Verification items for the finished model (mm, model axes). Coordinates: 2 decimals unless noted, no trailing zeros. Write each loop counter-clockwise with the first axis right and the second up, starting at its lowest first coordinate (ties: lowest second). Pieces come first, ordered by that corner, then holes. Notation, with made-up numbers: (49.25, 30.5) -> (106.25, 30.5) arc R20 ccw to (106.25, 59.5) -> close; hole circle Ø4 at (-18.75, -2.5). An arc over 180 degrees is marked (long way). Answer in a Markdown table with one row per item.
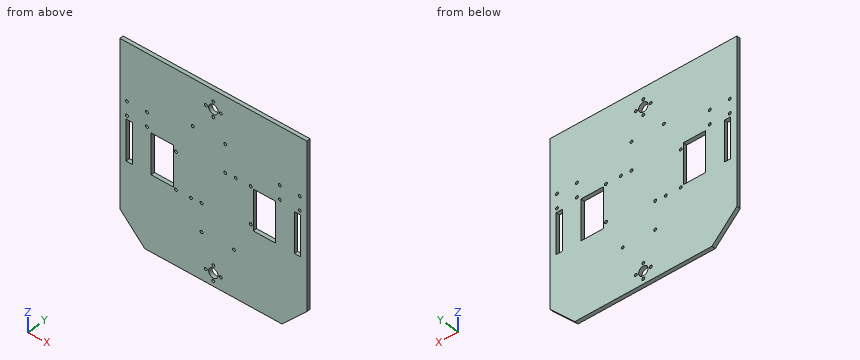
```python
from build123d import *

# Parameters (mm, degrees)
ESQUISSE1_R              = 7.5
ESQUISSE1_R_2            = 2.3
BOSS_EXTRU_1_DEPTH       = 6
ESQUISSE7_W              = 10
ESQUISSE7_H              = 64
ENL_V_MAT_EXTRU_9_DEPTH  = 10.5
ESQUISSE6_R              = 2.3
ENL_V_MAT_EXTRU_10_DEPTH = 50
ENL_V_MAT_EXTRU_11_DEPTH = 50
ESQUISSE11_R             = 2.3
ENL_V_MAT_EXTRU_15_DEPTH = 10


with BuildPart() as part:
    # Esquisse1 → Boss.-Extru.1 (new body)
    with BuildSketch(Plane(origin=(0, 0, 0), x_dir=(1, 0, 0), z_dir=(0, 1, 0))):
        Polygon((-150, 0), (-150, 260), (-110, 300), (110, 300), (150, 260), (150, 0), align=None)
        with Locations(Location((0, 30, 0), (0, 0, 270))):
            Circle(ESQUISSE1_R, mode=Mode.SUBTRACT)
        with Locations(Location((0, 18, 0), (0, 0, 270))):
            Circle(ESQUISSE1_R_2, mode=Mode.SUBTRACT)
        with Locations(Location((12, 30, 0), (0, 0, 270))):
            Circle(ESQUISSE1_R_2, mode=Mode.SUBTRACT)
        with Locations(Location((0, 42, 0), (0, 0, 270))):
            Circle(ESQUISSE1_R_2, mode=Mode.SUBTRACT)
        with Locations(Location((-12, 30, 0), (0, 0, 270))):
            Circle(ESQUISSE1_R_2, mode=Mode.SUBTRACT)
        with Locations(Location((0, 280, 0), (0, 0, 270))):
            Circle(ESQUISSE1_R, mode=Mode.SUBTRACT)
        with Locations(Location((-12, 280, 0), (0, 0, 270))):
            Circle(ESQUISSE1_R_2, mode=Mode.SUBTRACT)
        with Locations(Location((0, 268, 0), (0, 0, 270))):
            Circle(ESQUISSE1_R_2, mode=Mode.SUBTRACT)
        with Locations(Location((12, 280, 0), (0, 0, 270))):
            Circle(ESQUISSE1_R_2, mode=Mode.SUBTRACT)
        with Locations(Location((0, 292, 0), (0, 0, 270))):
            Circle(ESQUISSE1_R_2, mode=Mode.SUBTRACT)
    extrude(amount=BOSS_EXTRU_1_DEPTH)

    # Esquisse7 → Enlèv. mat.-Extru.9 (cut)
    with BuildSketch(Plane(origin=(0, 6, 0), x_dir=(1, 0, 0), z_dir=(0, 1, 0))):
        with Locations((-135, 150)):
            Rectangle(ESQUISSE7_W, ESQUISSE7_H)
    enl_v_mat_extru_9 = extrude(amount=-ENL_V_MAT_EXTRU_9_DEPTH, mode=Mode.SUBTRACT)

    # Esquisse6 → Enlèv. mat.-Extru.10 (cut)
    with BuildSketch(Plane(origin=(0, 6, 0), x_dir=(1, 0, 0), z_dir=(0, 1, 0))):
        with Locations(Location((-138.5, 90, 0), (0, 0, 270))):
            Circle(ESQUISSE6_R)
        with Locations(Location((-138.5, 112, 0), (0, 0, 270))):
            Circle(ESQUISSE6_R)
        with Locations(Location((-106.5, 112, 0), (0, 0, 270))):
            Circle(ESQUISSE6_R)
        with Locations(Location((-106.5, 90, 0), (0, 0, 270))):
            Circle(ESQUISSE6_R)
    enl_v_mat_extru_10 = extrude(amount=-ENL_V_MAT_EXTRU_10_DEPTH, mode=Mode.SUBTRACT)

    # Esquisse4 → Enlèv. mat.-Extru.11 (cut)
    with BuildSketch(Plane(origin=(0, 6, 0), x_dir=(1, 0, 0), z_dir=(0, 1, 0))):
        Polygon((-100, 150), (-100, 182), (-64, 182), (-64, 118), (-100, 118), align=None)
    enl_v_mat_extru_11 = extrude(amount=-ENL_V_MAT_EXTRU_11_DEPTH, mode=Mode.SUBTRACT)

    # Symétrie1: Enlèv. mat.-Extru.9 across plane
    add(enl_v_mat_extru_9.mirror(Plane(origin=(0, 0, 0), x_dir=(0, 0, 1), z_dir=(1, 0, 0))), mode=Mode.SUBTRACT)

    # Symétrie2: Enlèv. mat.-Extru.11 across plane
    add(enl_v_mat_extru_11.mirror(Plane(origin=(0, 0, 0), x_dir=(0, 0, 1), z_dir=(1, 0, 0))), mode=Mode.SUBTRACT)

    # Symétrie3: Enlèv. mat.-Extru.10 across plane
    add(enl_v_mat_extru_10.mirror(Plane(origin=(0, 0, 0), x_dir=(0, 0, 1), z_dir=(1, 0, 0))), mode=Mode.SUBTRACT)

    # Esquisse11 → Enlèv. mat.-Extru.15 (cut)
    with BuildSketch(Plane(origin=(0, 6, 0), x_dir=(1, 0, 0), z_dir=(0, 1, 0))):
        with Locations(Location((36, 116, 0), (0, 0, 270))):
            Circle(ESQUISSE11_R)
        with Locations(Location((60, 116, 0), (0, 0, 270))):
            Circle(ESQUISSE11_R)
        with Locations(Location((60, 174, 0), (0, 0, 270))):
            Circle(ESQUISSE11_R)
        with Locations(Location((-19, 227, 0), (0, 0, 270))):
            Circle(ESQUISSE11_R)
        with Locations(Location((-19, 183, 0), (0, 0, 270))):
            Circle(ESQUISSE11_R)
        with Locations(Location((33, 227, 0), (0, 0, 270))):
            Circle(ESQUISSE11_R)
        with Locations(Location((19, 117, 0), (0, 0, 270))):
            Circle(ESQUISSE11_R)
        with Locations(Location((19, 73, 0), (0, 0, 270))):
            Circle(ESQUISSE11_R)
        with Locations(Location((-33, 73, 0), (0, 0, 270))):
            Circle(ESQUISSE11_R)
        with Locations(Location((-60, 126, 0), (0, 0, 270))):
            Circle(ESQUISSE11_R)
        with Locations(Location((-36, 184, 0), (0, 0, 270))):
            Circle(ESQUISSE11_R)
        with Locations(Location((-60, 184, 0), (0, 0, 270))):
            Circle(ESQUISSE11_R)
    extrude(amount=-ENL_V_MAT_EXTRU_15_DEPTH, mode=Mode.SUBTRACT)


solid = part.part
```
1. Depth check by flat-ended pin: P1, Ø4, axis at x = 12, z = -280, coming from the -Y side. Enter the tip coordinate at first touch or a pass-through.
Geometry says:
| item | result |
|---|---|
| P1 | through |
2. Section check B-B, the plane y = 5.05. State how many separate pieces and enclosed holes the cut face has, plus the area to 3 significant figures.
Geometry says:
| item | result |
|---|---|
| separate pieces | 1 |
| enclosed holes | 34 |
| area | 81,700 mm^2 |
3. Thickness scan on line 1 (X direction, y = 1.75, z = -112); line 2 (X direction, y = 5.1, z = -169); line 3 (Z direction, x = -17.5, y = 3.7). Record the ranges inside material, lowest first. Write a range as from..to.
Geometry says:
| item | result |
|---|---|
| line 1 | -150..-140.8, -136.2..-108.8, -104.2..104.2, 108.8..136.2, 140.8..150 |
| line 2 | -150..-140, -130..-100, -64..64, 100..130, 140..150 |
| line 3 | -300..-228.74, -225.26..-184.74, -181.26..0 |
4. Section check A-A, the plane z = -134. Record the boundary of the cut face in (x, y), plus the area to 3 significant figures.
Geometry says:
| item | result |
|---|---|
| outline | (-150, 0) -> (-140, 0) -> (-140, 6) -> (-150, 6) -> close; (-130, 0) -> (-100, 0) -> (-100, 6) -> (-130, 6) -> close; (-64, 0) -> (64, 0) -> (64, 6) -> (-64, 6) -> close; (100, 0) -> (130, 0) -> (130, 6) -> (100, 6) -> close; (140, 0) -> (150, 0) -> (150, 6) -> (140, 6) -> close |
| area | 1,250 mm^2 |
